```python
from build123d import *

# Parameters (mm, degrees)
F1_DEPTH = 25.4
F0_W     = 31.75
F0_H     = 19.05
F2_DEPTH = 22.225
F3_SIZE  = 12.69999
F4_SIZE  = 9.52499


# Not quite as in the source:
# - a fillet or chamfer is up to 0.001 mm smaller than in the source, because OpenCascade refuses the exact size


with BuildPart() as f1:
    # F0 (on Top) → F1 (new body)
    with BuildSketch(Plane.XY):
        Polygon((0, 31.75), (0, 0), (25.4, 0), (25.4, 12.7), (25.4, 31.75), align=None)
    extrude(amount=F1_DEPTH)

    # F0 (on Top) → F2 (join)
    with BuildSketch(Plane.XY):
        Polygon((0, 31.75), (0, 0), (25.4, 0), (25.4, 12.7), (25.4, 31.75), align=None)
        with Locations((41.275, 22.225)):
            Rectangle(F0_W, F0_H)
    extrude(amount=F2_DEPTH)

    # F3 (size 12.7 in the source; OpenCascade refuses exactly that, so slightly less here)
    f3_edges = [f1.edges().sort_by_distance(p)[0] for p in [
        (25.4, 15.875, 25.4),
        (0, 15.875, 25.4),
    ]]
    chamfer(f3_edges, length=F3_SIZE)

    # F4 (size 9.525 in the source; OpenCascade refuses exactly that, so slightly less here)
    f4_edges = [f1.edges().sort_by_distance(p)[0] for p in [
        (36.512505, 12.7, 22.225),
        (36.512505, 31.75, 22.225),
    ]]
    chamfer(f4_edges, length=F4_SIZE)


solid = f1.part
```
Read the model definition and answer for the solid it produces. Units are mm, in the model's axes. A direction names the side the tool comes from. Coordinates: 2 decimals unless noted, no trailing zeros. Write each loop counter-clockwise with the first axis right and the second up, starting at its lowest first coordinate (ties: lowest second). Pieces come first, ordered by that corner, then holes. Notation, with made-up numbers: (-22.75, -3.75) - (6.25, -3.75) arc R19 ccw to (6.25, 16.25) - close; hole circle Ø9 at (1, 84). An arc over 180 degrees is marked (long way). Answer as a JSON object with one key per item and string values. Group by question number.
1. A cutting plane is placed at C-C (x = 12). Determine the outline of the cut face in (y, z), plus the area to 3 significant figures.
2. A cutting plane is placed at D-D (z = 19.25). Determine the outline of the cut face in (x, y).
3. A cutting plane is placed at B-B (z = 7.75). Determine the outline of the cut face in (x, y), plus the area to 3 significant figures.
4. Consider L1, parallel to X at y = 1, z = 7; L2, parallel to Y at x = 25.5, z = 9; L3, parallel to Z at x = 51, y = 27.5. Determine where each line is inside the solid, lowest interval first. Write a range as [from, to].
5. Which of the six approach directions +Z, -Z, +X, -X, +Y, -Y give full straight-line access (tool end or side, diameter ignored) to faces 1 (the flat face through (41, 12.7, 6)), 2 (the flat face through (41, 17, 17)), 3 (the flat face through (36.8, 26.92, 17.53))?
6. Each of these flat-tipped pins is pushed along its axis until it touches: P1, Ø2, axis at x = 18.5, z = 23, coming from the +Y side; P2, Ø14, axis at y = 3.5, z = 8.5, coming from the +X side; P3, Ø4, axis at x = 37, z = 8.5, coming from the -Y side. Where does it stop, or does it pass through?
Worked out:
{
 "1": {"outline": "(0, 0) - (31.75, 0) - (31.75, 24.7) - (0, 24.7) - close", "area": "784 mm²"},
 "2": {"outline": "(6.55, 0) - (18.85, 0) - (18.85, 19.25) - (57.15, 19.25) - (57.15, 25.2) - (18.85, 25.2) - (18.85, 31.75) - (6.55, 31.75) - close"},
 "3": {"outline": "(0, 0) - (25.4, 0) - (25.4, 12.7) - (57.15, 12.7) - (57.15, 31.75) - (0, 31.75) - close", "area": "1,410 mm²"},
 "4": {"L1": "x = [0, 25.4]", "L2": "y = [12.7, 31.75]", "L3": "z = [0, 16.95]"},
 "5": {"face 1": "+Z, -Z, +X, -Y", "face 2": "+Z, +X, -Y", "face 3": "+Z, +X, +Y"},
 "6": {"P1": "stops at y = 22.45", "P2": "stops at x = 25.4", "P3": "stops at y = 12.7"}
}
